Here's how the part is built. I have some questions about the finished solid (model axes, mm). A direction names the side the tool comes from. Coordinates: 2 decimals unless noted, no trailing zeros. Loops run counter-clockwise (first coordinate to the right, second up) from the corner with the lowest first, then second, coordinate; pieces in that order, holes last. Notation, with made-up numbers: M 24.5,59 L 74.5,59 A19 cw 74.5,91 Z; hole C 54.25,31.25 d10. An arc over 180 degrees is marked long. Use CSV: the item, a comma, the result in double quotes. Start each with the question number.
Q1. Which directions (+Z, -Z, +X, -X, +Y, -Y) give clear straight access to the entire face, cutting with the end or side of a thin tool? Please do faces 1 (the flat face through (9, 33.075, 4)), 2 (the cylindrical face through (1.426, -33.571, 3.676)), 3 (the flat face through (9, -31, 2)), 4 (the flat face through (49, -35.075, 4)), 5 (the flat face through (86, -33.075, 4)).
Q2. For pin 1 Ø2.5 at (x, y) = (85.81, -30.925) entering from -Z; pin 2 Ø2.5 at (x, z) = (9.31, 4.125) entering from -Y (3 decimals), each with a flat end and sliding along its axis, tell me the tip position at first contact or that it passes through.
Q3. If we mould it in two halves opening along Z, with no side actions, what happens to faces 6 (the flat face through (49, 0, 8.25)), 7 (the cylindrical face through (87.81, -30.84, 0.99)), 8 (the cylindrical face through (87.75, -34.09, 4.93))? For each: +Z half, -Z half, draft (parallel to the pull), parting line (faces both ways), or undercut.
Q4. If we section it at A-A (x = 9.31): Please give me the cut outline in (y, z) (3 decimals), and give its area (3 significant figures).
Q5. Please list where these lines run through material, in increasing order: probe 1 along Y at (x, z) = (9.31, 1) (3 decimals); probe 2 along X at (y, z) = (-29.5, 1.75); probe 3 along Z at (x, y) = (85.81, -33.8) (3 decimals). Write a range as [from, to].
from build123d import *

# Parameters (mm, degrees)
SKETCH2_W           = 100
SKETCH2_H           = 70.15
BOSS_EXTRUDE1_DEPTH = 8.25
FILLET1_R           = 5
CUT_EXTRUDE1_START  = -35.075
SKETCH3_R           = 2.1
CUT_EXTRUDE1_DEPTH  = 2
FILLET2_R           = 1
SKETCH4_R           = 2
CUT_EXTRUDE2_DEPTH  = 2


with BuildPart() as part:
    # Sketch2 → Boss-Extrude1 (new body)
    with BuildSketch(Plane.XY):
        with Locations((50, 0)):
            Rectangle(SKETCH2_W, SKETCH2_H)
    extrude(amount=BOSS_EXTRUDE1_DEPTH)

    # Fillet1
    fillet1_edges = [part.edges().sort_by_distance(p)[0] for p in [
        (0, 35.075, 4.125),
        (100, 35.075, 4.125),
        (100, -35.075, 4.125),
        (0, -35.075, 4.125),
    ]]
    fillet(fillet1_edges, radius=FILLET1_R)

    # Sketch3 → Cut-Extrude1 (cut)
    with BuildSketch(Plane(origin=(0, 0, 0), x_dir=(1, 0, 0), z_dir=(0, 1, 0)).offset(CUT_EXTRUDE1_START)):
        with Locations((9.31, -4.125)):
            Circle(SKETCH3_R)
        with Locations((85.81, -4.125)):
            Circle(SKETCH3_R)
    cut_extrude1 = extrude(amount=CUT_EXTRUDE1_DEPTH, mode=Mode.SUBTRACT)

    # Mirror1: Cut-Extrude1 across plane
    add(cut_extrude1.mirror(Plane.ZX), mode=Mode.SUBTRACT)

    # Fillet2
    fillet2_edges = [part.edges().sort_by_distance(p)[0] for p in [
        (100, 0, 8.25),
        (50, -35.075, 8.25),
        (0, 0, 8.25),
        (50, 35.075, 8.25),
        (1.464466094, 33.610533906, 8.25),
        (98.535533906, 33.610533906, 8.25),
        (1.464466094, -33.610533906, 8.25),
        (98.535533906, -33.610533906, 8.25),
    ]]
    fillet(fillet2_edges, radius=FILLET2_R)

    # Sketch4 → Cut-Extrude2 (cut)
    with BuildSketch(Plane.XY):
        with Locations((9.31, -30.925)):
            Circle(SKETCH4_R)
        with Locations((9.31, 30.925)):
            Circle(SKETCH4_R)
    cut_extrude2 = extrude(amount=CUT_EXTRUDE2_DEPTH, mode=Mode.SUBTRACT)

    # Mirror2: Cut-Extrude2 across plane
    add(cut_extrude2.mirror(Plane(origin=(47.56, 0, 0), x_dir=(0, 0, 1), z_dir=(1, 0, 0))), mode=Mode.SUBTRACT)


solid = part.part
Results below:
1,face 1,"+Y"
1,face 2,"+Z, -Z, -X, -Y"
1,face 3,"-Z"
1,face 4,"+Z, -Z, +X, -X, -Y"
1,face 5,"-Y"
2,pin 1,"z = 2"
2,pin 2,"y = -33.075"
3,face 6,"+Z half"
3,face 7,"draft"
3,face 8,"undercut"
4,outline,"M -35.075,0 L -32.925,0 L -32.925,2 L -28.925,2 L -28.925,0 L 28.925,0 L 28.925,2 L 32.925,2 L 32.925,0 L 35.075,0 L 35.075,2.025 L 33.075,2.025 L 33.075,6.225 L 35.075,6.225 L 35.075,7.25 A1 ccw 34.075,8.25 L -34.075,8.25 A1 ccw -35.075,7.25 L -35.075,6.225 L -33.075,6.225 L -33.075,2.025 L -35.075,2.025 Z"
4,area,"546 mm^2"
5,probe 1,"[-35.075, -32.925], [-28.925, 28.925], [32.925, 35.075]"
5,probe 2,"[0, 7.91], [10.71, 84.41], [87.21, 100]"
5,probe 3,"[0, 2.025], [6.225, 8.25]"
